Build history of the part. All positions in model axes, mm. A direction names the side the tool comes from. Give positions to 0.01 mm unless a question says otherwise; leave off trailing zeros. Write each loop counter-clockwise with the first axis right and the second up, starting at its lowest first coordinate (ties: lowest second). Pieces come first, ordered by that corner, then holes. Notation, with made-up numbers: M -34.5,-30 L -23.5,-30 A12 cw -23.5,-8 Z; hole C -5,-35.5 d11. An arc over 180 degrees is marked long. Return JSON: item names as keys, results as strings. Group by question number.
Q1. Band-saw the part on C-C, the plane x = 58.5. Give the cut face in (y, z).
Q2. Wall check: probe 1 along Y at (x, z) = (85, 32.5); probe 2 along X at (y, z) = (6, 10.5); probe 3 along X at (y, z) = (105, 8.5). Give the ranges that are in metal, low to high.
Q3. Band-saw the part on B-B, the plane y = 85. Give the cut face in (x, z).
Q4. Tool access for faces 1 (the flat face through (70, 37, 0)), 2 (the flat face through (103.523, 92, 20)), 3 (the flat face through (56, 34.23, 20)): list every direction of +Z, -Z, +X, -X, +Y, -Y with a clear straight run to the whole face (end or side of a thin tool).
Q5. Band-saw the part on A-A, the plane z = 31.5. Give the cut face in (x, y), then the cut area to 3 significant figures.
Q6. Flat gauge pins, fed straight in: pin 1 Ø20 at (x, z) = (64, 26.5) entering from -Y; pin 2 Ø6 at (y, z) = (9, 11) entering from +X; pin 3 Ø3 at (x, z) = (12.5, 8.5) entering from +Y. Where does each tip first touch, or does it go through?
from build123d import *

# Parameters (mm, degrees)
F1_DEPTH = 40


with BuildPart() as f1:
    # F0 (on Top) → F1 (new body)
    with BuildSketch(Plane.XY):
        with BuildLine():
            Line((0, 19.229688), (0, 0))
            Line((0, 0), (5, 0))
            Line((5, 0), (5, 19.229688))
            ThreePointArc((5, 19.229688), (9.393398, 29.836289), (20, 34.229688))
            Line((20, 34.229688), (93.523487, 34.229688))
            ThreePointArc((93.523487, 34.229688), (104.130089, 38.623086), (108.523487, 49.229688))
            Line((108.523487, 49.229688), (108.523487, 133.286635))
            Line((108.523487, 133.286635), (103.523487, 133.286635))
            Line((103.523487, 133.286635), (103.523487, 49.229688))
            ThreePointArc((103.523487, 49.229688), (100.594555, 42.15862), (93.523487, 39.229688))
            Line((93.523487, 39.229688), (20, 39.229688))
            ThreePointArc((20, 39.229688), (5.857864, 33.371823), (0, 19.229688))
        make_face()
    extrude(amount=F1_DEPTH)


solid = f1.part
From the geometry:
{
 "1": {"outline": "M 34.23,0 L 39.23,0 L 39.23,40 L 34.23,40 Z"},
 "2": {"probe 1": "y = 34.23 to 39.23", "probe 2": "x = 0 to 5", "probe 3": "x = 103.52 to 108.52"},
 "3": {"outline": "M 103.52,0 L 108.52,0 L 108.52,40 L 103.52,40 Z"},
 "4": {"face 1": "-Z, +X, -X, +Y, -Y", "face 2": "+Z, -Z, -X, +Y", "face 3": "+Z, -Z, +X, -Y"},
 "5": {"outline": "M 0,0 L 5,0 L 5,19.23 A15 cw 20,34.23 L 93.52,34.23 A15 ccw 108.52,49.23 L 108.52,133.29 L 103.52,133.29 L 103.52,49.23 A10 cw 93.52,39.23 L 20,39.23 A20 ccw 0,19.23 Z", "area": "1,120 mm^2"},
 "6": {"pin 1": "stops at y = 34.23", "pin 2": "stops at x = 5", "pin 3": "stops at y = 38.31"}
}
